```python
from build123d import *

# Parameters (mm, degrees)
SKETCH_1_R          = 62.989422777
EXTRUDE_1_DEPTH     = 10
SKETCH_2_W          = 30.2
SKETCH_2_H          = 25.2
CUT_EXTRUDE_1_DEPTH = 5


with BuildPart() as part:
    # 草图1 → 凸台-拉伸1 (new body)
    with BuildSketch(Plane(origin=(0, 0, 0), x_dir=(1, 0, 0), z_dir=(0, 1, 0))):
        with Locations(Location((0, 0, 0), (0, 0, 270))):
            Circle(SKETCH_1_R)
    extrude(amount=EXTRUDE_1_DEPTH)

    # 草图2 → 切除-拉伸1 (cut)
    with BuildSketch(Plane(origin=(0, 10, 0), x_dir=(1, 0, 0), z_dir=(0, 1, 0))):
        with Locations((-32, 0)):
            Rectangle(SKETCH_2_W, SKETCH_2_H)
        with Locations((32, 0)):
            Rectangle(SKETCH_2_W, SKETCH_2_H)
    extrude(amount=-CUT_EXTRUDE_1_DEPTH, mode=Mode.SUBTRACT)


solid = part.part
```
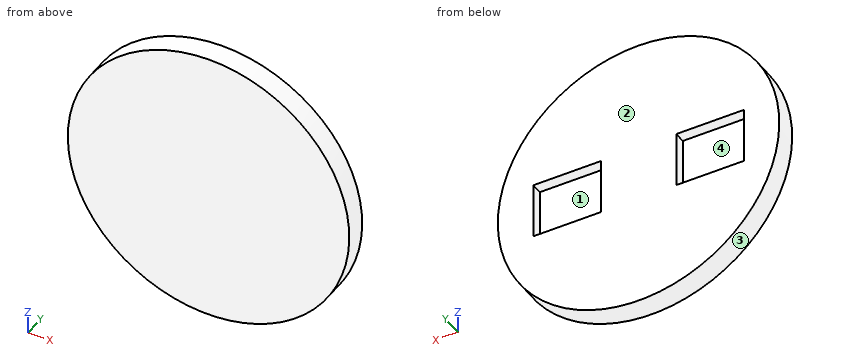
Model file for the job. Use its own axes, mm. Face numbers are marked on the shaded views. Round coordinates to 2 decimals unless told otherwise and drop trailing zeros. Order: outer loops, then holes, each group sorted by start corner. A loop starts at its lowest first (then second) coordinate and runs counter-clockwise, first axis right, second up. Notation, with made-up numbers: (83, 5.25) -> (103, 5.25) arc R10 ccw to (103, 14.25) -> close; hole circle Ø6 at (-35.5, 22.25). An arc over 180 degrees is marked (long way). Use one line per item in the form item = value.
Item 1: Pull direction X, two halves, no side cores. Call the marked faces 1, 2, 3 and 4: released by +X, released by -X, zero draft, split by the parting line, or undercut.
Returned:
face_1 = undercut
face_2 = zero draft
face_3 = split by the parting line
face_4 = undercut
Item 2: Flat gauge pins, fed straight in: pin 1 Ø1.5 at (y, z) = (1.5, -13) entering from +X; pin 2 Ø1.5 at (x, y) = (-35, 7.5) entering from -Z; pin 3 Ø2.5 at (x, y) = (-27.5, 8) entering from +Z. Where does each tip first touch, or does it go through?
Returned:
pin_1 = 61.79
pin_2 = -52.86
pin_3 = 57.26
Item 3: Cut at B-B, the plane y = 1.75. Write the cut outline in (x, z), and give its area (3 significant figures).
Returned:
outline = circle Ø125.98 at (0, 0)
area = 12,500 mm^2
Item 4: Cut at C-C, the plane x = 43.5. Write the cut outline in (y, z).
Returned:
outline = (0, -45.56) -> (10, -45.56) -> (10, -12.6) -> (5, -12.6) -> (5, 12.6) -> (10, 12.6) -> (10, 45.56) -> (0, 45.56) -> close
Item 5: Cut at A-A, the plane z = 0. Write the cut outline in (x, y).
Returned:
outline = (-62.99, 0) -> (62.99, 0) -> (62.99, 10) -> (47.1, 10) -> (47.1, 5) -> (16.9, 5) -> (16.9, 10) -> (-16.9, 10) -> (-16.9, 5) -> (-47.1, 5) -> (-47.1, 10) -> (-62.99, 10) -> close
Item 6: Cut at D-D, the plane x = -27. Write the cut outline in (y, z).
Returned:
outline = (0, -56.91) -> (10, -56.91) -> (10, -12.6) -> (5, -12.6) -> (5, 12.6) -> (10, 12.6) -> (10, 56.91) -> (0, 56.91) -> close
Item 7: Drill centre lines: line 1 (X direction, y = 8.25, z = -1.5); line 2 (Y direction, x = -37, z = 8); line 3 (X direction, y = 9.25, z = 10.5). Where is each one in solid material? Low to high.
Returned:
line_1 = -62.97 to -47.1, -16.9 to 16.9, 47.1 to 62.97
line_2 = 0 to 5
line_3 = -62.11 to -47.1, -16.9 to 16.9, 47.1 to 62.11
